Autodesk Inventor part; units mm, degrees
ref_plane "YZ Plane" through (0, 0, 0) normal (1, 0, 0) x (0, 1, 0)
ref_plane "XZ Plane" through (0, 0, 0) normal (0, 1, 0) x (-1, 0, 0)
ref_plane "XY Plane" through (0, 0, 0) normal (0, 0, 1) x (1, 0, 0)
sketch "Szkic1" plane through (0, 0, 0) normal (1, 0, 0) x (0, 1, 0)
  circle A0 centre (0, 0) radius 6.5
  circle A1 centre (0, 0) radius 1.75
  line L0 (0, 1.75) -> (0, -1.0846)
  line L1 (-1, 1.9718) -> (-1, -1.0846)
  line L2 (8, 0) -> (-8, 0)
  line L3 (-8, 0) -> (-8, -1)
  line L4 (-8, -1) -> (8, -1)
  line L5 (8, -1) -> (8, 0)
  line L6 (8, 0) -> (-8, 0)
  line L7 (-8, 0) -> (-8, 1)
  line L8 (-8, 1) -> (8, 1)
  line L9 (8, 1) -> (8, 0)
  line L10 (0, 8) -> (1, 8)
  line L11 (1, 8) -> (1, -8)
  line L12 (1, -8) -> (0, -8)
  line L13 (0, 8) -> (-1, 8)
  line L14 (-1, 8) -> (-1, -8)
  line L15 (-1, -8) -> (0, -8)
  line L16 (0, -8) -> (0, 8)
  point P0 (-1, -1.4361)
  point P1 (-1, 1.4361)
  point P2 (-6.4226, -1)
  point P3 (-6.4226, 1)
  point P4 (1, -6.4226)
  point P5 (-1, -6.4226)
  point P6 (6.4226, 1)
  point P7 (6.4226, -1)
  point P8 (-1, 6.4226)
  point P9 (1, 6.4226)
  dimension "d1" = 3.5
  dimension "d0" = 13
  dimension "d2" = 1
  dimension "d14" = 16
  dimension "d16" = 16
  dimension "d18" = 2
  dimension "d19" = 2
sketch "Szkic2" plane through (0, 0, 0) normal (0, 0, 1) x (1, 0, 0)
  line L0 (0, 0) -> (5, 0)
  line L1 (5, 0) -> (5, 6)
  line L2 (5, 6) -> (0, 6)
  line L3 (0, 6) -> (0, 0)
  line L4 (0, 0) -> (-5, 0)
  line L5 (-5, 0) -> (-5, 6)
  line L6 (-5, 6) -> (0, 6)
  line L7 (0, 6) -> (0, 0)
  line L8 (0, 0) -> (5, 0)
  line L9 (5, 0) -> (5, -6)
  line L10 (5, -6) -> (0, -6)
  line L11 (0, -6) -> (0, 0)
  line L12 (0, 0) -> (-5, 0)
  line L13 (-5, 0) -> (-5, -6)
  line L14 (-5, -6) -> (0, -6)
  line L15 (0, -6) -> (0, 0)
  line L16 (5, 6) -> (4, 6)
  line L17 (4, 6) -> (4, 8)
  line L18 (4, 8) -> (5, 8)
  line L19 (5, 8) -> (5, 6)
  line L20 (2, 6) -> (1, 6)
  line L21 (1, 6) -> (1, 8)
  line L22 (1, 8) -> (2, 8)
  line L23 (2, 8) -> (2, 6)
  line L24 (-5, 6) -> (-4, 6)
  line L25 (-4, 6) -> (-4, 8)
  line L26 (-4, 8) -> (-5, 8)
  line L27 (-5, 8) -> (-5, 6)
  line L28 (-2, 6) -> (-1, 6)
  line L29 (-1, 6) -> (-1, 8)
  line L30 (-1, 8) -> (-2, 8)
  line L31 (-2, 8) -> (-2, 6)
  point P0 (-1, 6)
  point P1 (1, 6)
  point P2 (0, 6)
  dimension "d3" = 5
  dimension "d4" = 6
  dimension "d5" = 10
  dimension "d6" = 12
  dimension "d7" = 1
  dimension "d8" = 2
  dimension "d9" = 1
  dimension "d10" = 1
  dimension "d11" = 2
  dimension "d12" = 1
  dimension "d13" = 2
extrude "Wyciągnięcie proste1" add sketch "Szkic1" along normal mid plane 10 contours L2 A1 L8 A0 | A0 L4 A1 L2 | L8 A1 L11 A0 | A0 L11 A1 L4 | L11 A1 L16 A0 | A0 L16 A1 L11 | L16 A1 L1 L14 A0 | A0 L14 A1 L16 | L14 L1 A1 L8 A0 | A0 L4 A1 L14 | L2 A1 L8 L1 | L1 L4 A1 L2 | L8 A1 L2 A0 | L1 L8 A1 | A0 L2 A1 L4 | A1 L4 L1 L14
extrude "Wyciągnięcie proste2" add sketch "Szkic1" along normal mid plane 2 contours L2 L5 L4 A0 | A0 L8 L9 L2 | A0 L16 L10 L11 | L11 L12 L16 A0 | A0 L14 L13 L16 | L16 L15 L14 A0 | A0 L2 L7 L8 | L4 L3 L2 A0
revolve "Obrót1" add sketch "Szkic2" angle 360 about axis through (0, 0, 0) along (1, 0, 0) contours L2 L17 L18 L19 | L21 L22 L23 L2 | L6 L31 L30 L29 | L27 L26 L25 L6
sketch "Sketch3" plane through (-5, 0, 0) normal (-1, 0, 0) x (0, 0, 1)
  circle A0 centre (0, 0) radius 3.5355
  point P0 (2.4008, 2.5954)
  point P1 (-2.5954, 2.4008)
  point P2 (-2.4008, -2.5954)
  point P3 (2.5954, -2.4008)
  dimension "d25" = 7.071
  dimension "d28" = 360
hole "Hole2" at (-5, 2.5954, 2.4008) at (-5, 2.4008, -2.5954) at (-5, -2.5954, -2.4008) at (-5, -2.4008, 2.5954) direction (1, 0, 0) diameter 1.5 depth 2
sketch "Szkic4" plane through (1, 6.4226, -1) normal (-1, 0, 0) x (0, 0, 1)
  circle A0 centre (-4.605, -1.8752) radius 0.479
  circle A1 centre (-3.0498, -0.4418) radius 0.479
  circle A2 centre (-0.9626, 0.445) radius 0.479
  circle A3 centre (-5.8399, -4.0395) radius 0.479
  circle A4 centre (3.2445, 0.3734) radius 0.479
  circle A5 centre (5.4171, -0.7585) radius 0.479
  circle A6 centre (7.0233, -2.4367) radius 0.479
  circle A7 centre (7.9555, -4.5185) radius 0.479
  circle A8 centre (7.9555, -8.7018) radius 0.479
  circle A9 centre (6.6895, -10.7659) radius 0.479
  circle A10 centre (5.147, -12.2513) radius 0.479
  circle A11 centre (3.2445, -13.1654) radius 0.479
  circle A12 centre (-1.1045, -13.3006) radius 0.479
  circle A13 centre (-3.0498, -12.4071) radius 0.479
  circle A14 centre (-5.5022, -9.1808) radius 0.479
  circle A15 centre (-4.605, -10.9821) radius 0.479
  point P0 (1, -6.4226)
extrude "Wyciągnięcie proste3" cut sketch "Szkic4" against normal blind 0.5
sketch "Szkic5" plane through (-1, 6.4226, 1) normal (1, 0, 0) x (0, 0, -1)
  circle A0 centre (-5.8399, -4.0395) radius 0.479
  circle A1 centre (-4.801, -2.132) radius 0.479
  circle A2 centre (-3.3616, -0.7148) radius 0.479
  circle A3 centre (-1.5017, 0.4249) radius 0.479
  circle A4 centre (2.8454, 0.6357) radius 0.479
  circle A5 centre (4.8692, -0.2358) radius 0.479
  circle A6 centre (6.5094, -1.8534) radius 0.479
  circle A7 centre (7.6213, -3.7767) radius 0.479
  circle A8 centre (7.8771, -8.6528) radius 0.479
  circle A9 centre (6.8617, -10.6883) radius 0.479
  circle A10 centre (5.1318, -12.328) radius 0.479
  circle A11 centre (3.1684, -13.2494) radius 0.479
  circle A12 centre (-1.5017, -13.2494) radius 0.479
  circle A13 centre (-3.3616, -12.328) radius 0.479
  circle A14 centre (-4.9725, -10.6883) radius 0.479
  circle A15 centre (-5.8399, -8.6528) radius 0.479
  point P0 (1, -6.4226)
extrude "Wyciągnięcie proste4" cut sketch "Szkic5" against normal blind 0.5
properties part number "Poprawione_koło"
Could you check a few things on this model? Use its own coordinates, in mm. A direction names the side the tool comes from. Round coordinates to 2 decimals unless told otherwise and drop trailing zeros. Order: outer loops, then holes, each group sorted by start corner. A loop starts at its lowest first (then second) coordinate and runs counter-clockwise, first axis right, second up.
Q1. Imagine slicing it at B-B, the plane z = -6.75. State how many separate pieces and enclosed holes the cut face has, then the cut area to 3 significant figures.
Geometry says:
separate pieces: 3
enclosed holes: 0
area: 36.5 mm2
Q2. Which directions (+Z, -Z, +X, -X, +Y, -Y) give clear straight access to the entire face, cutting with the end or side of a thin tool? Please do faces 1 (the face through (-5, 0, 2)), 2 (the face through (0, -7, -1)), 3 (the face through (-3, -3, -2)), 4 (the face through (1.246, -5.354, 4.085)).
Geometry says:
face 1: +Z, -Z, -X, +Y, -Y
face 2: -Z, -Y
face 3: -X
face 4: none
Q3. Thinking about a two-plate mould opening in X: for faces 5 (the face through (1.25, -5.58, -3.79)), 6 (the face through (-4.51, -1.73, 7.81)), 7 (the face through (1.5, 6, -4)), 8 (the face through (-3, 3, 2)), which applies, released by +X, released by -X, zero draft, split by the parting line, or undercut?
Geometry says:
face 5: undercut
face 6: zero draft
face 7: undercut
face 8: released by -X
Q4. Imagine slicing it at C-C, the plane x = 3.25. List the corners of the cut face in (y, z) for me.
Geometry says:
outline: circle Ø13 at (0, 0); hole (-1, -1.44) arc R1.75 ccw (long way) to (-1, 1.44) - close
Q5. Imagine slicing it at A-A, the plane x = -3.5. List the corners of the cut face in (y, z) for me, then the cut area to 3 significant figures.
Geometry says:
outline: circle Ø13 at (0, 0); hole circle Ø1.5 at (-2.6, -2.4); hole circle Ø1.5 at (-2.4, 2.6); hole (-1, -1.44) arc R1.75 ccw (long way) to (-1, 1.44) - close; hole circle Ø1.5 at (2.4, -2.6); hole circle Ø1.5 at (2.6, 2.4)
area: 118 mm2
Q6. Please list where these lines run through material, in increasing order: probe 1 along X at (y, z) = (4.25, 5.5); probe 2 along X at (y, z) = (-4.25, -5.75); probe 3 along Y at (x, z) = (2.5, 1).
Geometry says:
probe 1: x = -5 to -4, -2 to -1.5, 1 to 2, 4 to 5
probe 2: x = -5 to -4, -2 to -1.5, 1.5 to 2, 4 to 5
probe 3: y = -6.42 to -1, 1.44 to 6.42
Q7. I'm going to push flat-ended pins straight in: P1, Ø0.8, axis at x = 0.5, y = 7, coming from the -Z side; P2, Ø2, axis at x = 1, z = -6, coming from the -Y side (3 decimals); P3, Ø5, axis at y = 0, z = 1, coming from the -X side. Where does each tip first touch, or does it pass through?
Geometry says:
P1: stops at z = -1
P2: stops at y = -6.245
P3: stops at x = -5
